Here's how the part is built. I have some questions about the finished solid (model axes, mm). Round coordinates to 2 decimals unless told otherwise and drop trailing zeros. Order: outer loops, then holes, each group sorted by start corner. A loop starts at its lowest first (then second) coordinate and runs counter-clockwise, first axis right, second up.
```python
from build123d import *

# Parameters (mm, degrees)
SKETCH1_R            = 27.5
SKETCH1_R_2          = 14.5
SKETCH1_R_3          = 1.5
BOSS_EXTRUDE1_DEPTH  = 3
CUT_EXTRUDE1_START   = -10
CUT_EXTRUDE1_DEPTH   = 10
M3_CLEARANCE_HOLE1_D = 3.6


with BuildPart() as part:
    # Sketch1 → Boss-Extrude1 (new body)
    with BuildSketch(Plane.XY):
        Circle(SKETCH1_R)
        Circle(SKETCH1_R_2, mode=Mode.SUBTRACT)
        with Locations((0, 22.5)):
            Circle(SKETCH1_R_3, mode=Mode.SUBTRACT)
        with Locations((22.5, 0)):
            Circle(SKETCH1_R_3, mode=Mode.SUBTRACT)
        with Locations((0, -22.5)):
            Circle(SKETCH1_R_3, mode=Mode.SUBTRACT)
        with Locations((-22.5, 0)):
            Circle(SKETCH1_R_3, mode=Mode.SUBTRACT)
    extrude(amount=BOSS_EXTRUDE1_DEPTH)

    # Sketch2 → Cut-Extrude1 (cut)
    with BuildSketch(Plane.XY.offset(3).offset(CUT_EXTRUDE1_START)):
        with BuildLine():
            ThreePointArc((-2.155688811, 27.415379001), (-19.445436483, 19.445436483), (-27.415379001, 2.155688811))
            Line((-27.415379001, 2.155688811), (-2.155688811, 27.415379001))
        make_face()
        with BuildLine():
            ThreePointArc((27.415379001, 2.155688811), (19.445436483, 19.445436483), (2.155688811, 27.415379001))
            Line((2.155688811, 27.415379001), (27.415379001, 2.155688811))
        make_face()
        with BuildLine():
            Line((27.415379001, -2.155688811), (2.155688811, -27.415379001))
            ThreePointArc((2.155688811, -27.415379001), (19.445436483, -19.445436483), (27.415379001, -2.155688811))
        make_face()
        with BuildLine():
            Line((-2.155688811, -27.415379001), (-27.415379001, -2.155688811))
            ThreePointArc((-27.415379001, -2.155688811), (-19.445436483, -19.445436483), (-2.155688811, -27.415379001))
        make_face()
    extrude(amount=CUT_EXTRUDE1_DEPTH, mode=Mode.SUBTRACT)

    # M3 Clearance Hole1 (through all)
    with Locations(Plane.XY.offset(3)):
        with Locations((0, 22.5), (-22.5, 0), (0, -22.5), (22.5, 0)):
            Hole(M3_CLEARANCE_HOLE1_D / 2)


solid = part.part
```
1) I need wall thicknesses on line 1 (Y direction, x = 0, z = 0.7); line 2 (X direction, y = 7, z = 0.5); line 3 (Y direction, x = -22.5, z = 2.4). Which ranges of each line are inside material? Lowest first, please.
2) If we section it at B-B (z = 1.6): Write out the boundary of the cut face in (x, y).
3) If we section it at A-A (y = 0): Write out the boundary of the cut face in (x, z).
4) We'd pull the mould along X, two halves only. Please class faces 1 (the flat face through (-6, -14, 3)), 2 (the flat face through (14.61, 14.96, 1.48)), 3 (the cylindrical face through (20.783, 0.541, 1.479)), 4 (the cylindrical face through (0, -27.5, 1.5)): +X half, -X half, draft (parallel to the pull), parting line (faces both ways), or undercut.
5) If we section it at D-D (x = -22.5): Write out the boundary of the cut face in (y, z), plus the area to 3 significant figures.
Solutions:
1. line 1: y = -27.5 to -24.3, -20.7 to -14.5, 14.5 to 20.7, 24.3 to 27.5
1. line 2: x = -22.57 to -12.7, 12.7 to 22.57
1. line 3: y = -7.07 to -1.8, 1.8 to 7.07
2. outline: (-27.42, -2.16) - (-2.16, -27.42) arc R27.5 ccw to (2.16, -27.42) - (27.42, -2.16) arc R27.5 ccw to (27.42, 2.16) - (2.16, 27.42) arc R27.5 ccw to (-2.16, 27.42) - (-27.42, 2.16) arc R27.5 ccw to start; hole circle Ø3.6 at (-22.5, 0); hole circle Ø29 at (0, 0); hole circle Ø3.6 at (0, -22.5); hole circle Ø3.6 at (0, 22.5); hole circle Ø3.6 at (22.5, 0)
3. outline: (-27.5, 0) - (-24.3, 0) - (-24.3, 3) - (-27.5, 3) - close; (-20.7, 0) - (-14.5, 0) - (-14.5, 3) - (-20.7, 3) - close; (14.5, 0) - (20.7, 0) - (20.7, 3) - (14.5, 3) - close; (24.3, 0) - (27.5, 0) - (27.5, 3) - (24.3, 3) - close
4. face 1: draft
4. face 2: +X half
4. face 3: undercut
4. face 4: parting line
5. outline: (-7.07, 0) - (-1.8, 0) - (-1.8, 3) - (-7.07, 3) - close; (1.8, 0) - (7.07, 0) - (7.07, 3) - (1.8, 3) - close
5. area: 31.6 mm2
